from build123d import *
from build123d.topology import SkipClean

# Parameters (mm, degrees)
SKETCH1_W           = 16
SKETCH1_H           = 3
BOSS_EXTRUDE1_DEPTH = 15
SKETCH2_R           = 1.282586005
CUT_EXTRUDE1_DEPTH  = 12
SKETCH3_R           = 4
BOSS_EXTRUDE2_DEPTH = 43


with BuildPart() as part:
    # Sketch1 → Boss-Extrude1 (new body)
    with BuildSketch(Plane.XY):
        with Locations((0, 21.58414062)):
            Rectangle(SKETCH1_W, SKETCH1_H)
    extrude(amount=BOSS_EXTRUDE1_DEPTH)

    # Sketch2 → Cut-Extrude1 (cut)
    with BuildSketch(Plane(origin=(0, 23.08414062, 0), x_dir=(1, 0, 0), z_dir=(0, 1, 0))):
        with Locations(Location((5, -6, 0), (0, 0, 270))):
            Circle(SKETCH2_R)
        with Locations(Location((-5, -6, 0), (0, 0, 270))):
            Circle(SKETCH2_R)
    extrude(amount=-CUT_EXTRUDE1_DEPTH, mode=Mode.SUBTRACT)

    # Sketch3 → Boss-Extrude2 (add)
    with BuildSketch(Plane(origin=(0, 23.08414062, 0), x_dir=(1, 0, 0), z_dir=(0, 1, 0))):
        with Locations(Location((0, -10.092270702, 0), (0, 0, 90))):
            Circle(SKETCH3_R)
    extrude(amount=BOSS_EXTRUDE2_DEPTH)

    # Sketch5 → Revolve1 (revolve)
    with SkipClean():  # the faces are left unmerged after this step: merging them gives an invalid solid
        with BuildSketch(Plane(origin=(0, 66.08414062, 0), x_dir=(1, 0, 0), z_dir=(0, 1, 0))):
            with BuildLine():
                ThreePointArc((4, -10.092270702), (2.828427125, -7.263843577), (0, -6.092270702))
                Line((0, -6.092270702), (0, -14.092270702))
                ThreePointArc((0, -14.092270702), (2.828427125, -12.920697827), (4, -10.092270702))
            make_face()
            with BuildLine():
                Line((0, -14.092270702), (0, -6.092270702))
                ThreePointArc((0, -6.092270702), (-4, -10.092270702), (0, -14.092270702))
            make_face()
        revolve(axis=Axis((0, 66.08414062, 6.092270702), (0, 0, 1)))


solid = part.part
Here's how the part is built. I have some questions about the finished solid (model axes, mm). A direction names the side the tool comes from. Round coordinates to 2 decimals unless told otherwise and drop trailing zeros. Loops run counter-clockwise (first coordinate to the right, second up) from the corner with the lowest first, then second, coordinate; pieces in that order, holes last.
1. If we section it at A-A on x = -5: Write out the boundary of the cut face in (y, z).
Answer list:
outline: (20.08, 0) - (23.08, 0) - (23.08, 4.72) - (20.08, 4.72) - close; (20.08, 7.28) - (23.08, 7.28) - (23.08, 15) - (20.08, 15) - close
2. If I drill on line 1 along X through (y, z) = (22.55, 6); line 2 along Y through (x, z) = (4.5, 2.5); line 3 along X through (y, z) = (26.5, 7.25), over which ranges is the centre line in solid material (lowest first)?
Answer list:
line 1: x = -8 to -6.28, -3.72 to 3.72, 6.28 to 8
line 2: y = 20.08 to 23.08
line 3: x = -2.81 to 2.81
3. Which directions (+Z, -Z, +X, -X, +Y, -Y) give clear straight access to the entire face, cutting with the end or side of a thin tool? Please do faces 1 (the face through (0, 20.084, 7)), 2 (the face through (2.43, 44.28, 13.27)).
Answer list:
face 1: +Z, -Z, +X, -X, -Y
face 2: +Y
4. For P1, Ø2.5, axis at x = -5, z = 6, coming from the +Y side; P2, Ø6, axis at x = 0, y = 29, coming from the -Z side; P3, Ø6, axis at y = 28, z = 7, coming from the -X side; P4, Ø6, axis at y = 46, z = 10.5, coming from the +X side, each with a flat end and sliding along its axis, tell me the tip position at first contact or that it passes through.
Answer list:
P1: passes through
P2: stops at z = 6.09
P3: stops at x = -4
P4: stops at x = 4
5. If we section it at B-B on x = 0: Write out the boundary of the cut face in (y, z), plus the area to 3 significant figures.
Answer list:
outline: (20.08, 0) - (23.08, 0) - (23.08, 6.09) - (66.08, 6.09) arc R4 ccw to (66.08, 14.09) - (23.08, 14.09) - (23.08, 15) - (20.08, 15) - close
area: 414 mm2
6. If we section it at C-C on z = 12.5: Write out the boundary of the cut face in (x, y), plus the area to 3 significant figures.
Answer list:
outline: (-8, 20.08) - (8, 20.08) - (8, 23.08) - (3.19, 23.08) - (3.19, 66.08) arc R3.19 ccw to (-3.19, 66.08) - (-3.19, 23.08) - (-8, 23.08) - close
area: 339 mm2
7. If we section it at D-D on y = 56: Write out the boundary of the cut face in (x, z), plus the area to 3 significant figures.
Answer list:
outline: circle Ø8 at (0, 10.09)
area: 50.3 mm2
